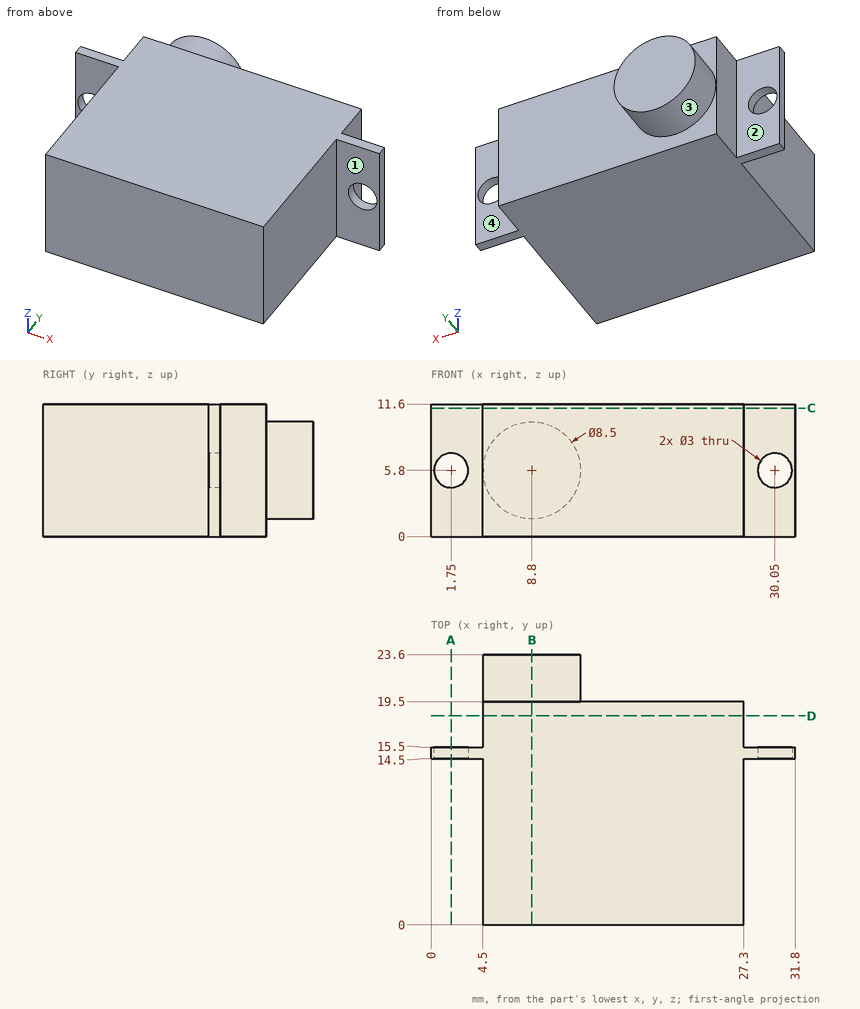
Source: three-view drawing plus pictorial views. Frame: mm from the lowest corner of the part. A direction names the side the tool comes from. Coordinates: 2 decimals unless noted, no trailing zeros. Order: outer loops, then holes, each group sorted by start corner. A loop starts at its lowest first (then second) coordinate and runs counter-clockwise, first axis right, second up.
1) Section A-A (x = 1.75). Return loops of the section in (y, z), then the cut area to 3 significant figures.
Result sheet:
outline: (14.5, 0) - (15.5, 0) - (15.5, 4.3) - (14.5, 4.3) - close; (14.5, 7.3) - (15.5, 7.3) - (15.5, 11.6) - (14.5, 11.6) - close
area: 8.60 mm2
2) Ray query, probe 1 along X at (y, z) = (15.1, 5.8); probe 2 along Z at (x, y) = (30.05, 15.15); probe 3 along Y at (x, z) = (16, 6.75). Return the intervals inside material, ascending.
Result sheet:
probe 1: x = 0 to 0.25, 3.25 to 28.55, 31.55 to 31.8
probe 2: z = 0 to 4.3, 7.3 to 11.6
probe 3: y = 0 to 19.5
3) Section C-C (z = 11.25). Return loops of the section in (x, y), then the cut area to 3 significant figures.
Result sheet:
outline: (0, 14.5) - (4.5, 14.5) - (4.5, 0) - (27.3, 0) - (27.3, 14.5) - (31.8, 14.5) - (31.8, 15.5) - (27.3, 15.5) - (27.3, 19.5) - (4.5, 19.5) - (4.5, 15.5) - (0, 15.5) - close
area: 454 mm2
4) First-contact query: P1, Ø5, axis at y = 3, z = 1, coming from the +X side; P2, Ø2, axis at x = 30.5, z = 5, coming from the +Y side; P3, Ø1, axis at x = 19, z = 3, coming from the +Y side; P4, Ø2, axis at x = 17, z = 4.5, coming from the -Y side. Flat tips, straight axial feed; report the tip coordinate or a pass-through.
Result sheet:
P1: stops at x = 27.3
P2: stops at y = 15.5
P3: stops at y = 19.5
P4: stops at y = 0
5) Section D-D (y = 18.25). Return loops of the section in (x, z), then the cut area to 3 significant figures.
Result sheet:
outline: (4.5, 0) - (27.3, 0) - (27.3, 11.6) - (4.5, 11.6) - close
area: 264 mm2
6) Set-up query: the marked faces 1, 2, 3 and 4. Return all of +Z, -Z, +X, -X, +Y, -Y with unobstructed straight access to the full face (end or side cutting, diameter ignored); none if empty.
Result sheet:
face 1: +Z, -Z, +X, -Y
face 2: +Z, -Z, -X, +Y
face 3: +Y
face 4: +Z, -Z, +X, +Y
7) Section B-B (x = 8.8). Return loops of the section in (y, z), then the cut area to 3 significant figures.
Result sheet:
outline: (0, 0) - (19.5, 0) - (19.5, 1.55) - (23.6, 1.55) - (23.6, 10.05) - (19.5, 10.05) - (19.5, 11.6) - (0, 11.6) - close
area: 261 mm2
